```python
from build123d import *

# Parameters (mm, degrees)
F0_W     = 71
F0_H     = 7.4
F0_R     = 3
F1_DEPTH = 3.95
F0_R_2   = 2.499
F2_DEPTH = 2.95
F3_R     = 3.69999


# Not quite as in the source:
# - a fillet or chamfer is up to 0.001 mm smaller than in the source, because OpenCascade refuses the exact size


with BuildPart() as f1:
    # F0 (on Front) → F1 (new body, symmetric)
    with BuildSketch(Plane.XZ):
        Rectangle(F0_W, F0_H)
        with Locations((-32, 0)):
            Circle(F0_R, mode=Mode.SUBTRACT)
        with Locations((-24, 0)):
            Circle(F0_R, mode=Mode.SUBTRACT)
        with Locations((-16, 0)):
            Circle(F0_R, mode=Mode.SUBTRACT)
        with Locations((-8, 0)):
            Circle(F0_R, mode=Mode.SUBTRACT)
        Circle(F0_R, mode=Mode.SUBTRACT)
        with Locations((8, 0)):
            Circle(F0_R, mode=Mode.SUBTRACT)
        with Locations((16, 0)):
            Circle(F0_R, mode=Mode.SUBTRACT)
        with Locations((24, 0)):
            Circle(F0_R, mode=Mode.SUBTRACT)
        with Locations((32, 0)):
            Circle(F0_R, mode=Mode.SUBTRACT)
    extrude(amount=F1_DEPTH, both=True)

    # F0 (on Front) → F2 (join, symmetric)
    with BuildSketch(Plane.XZ):
        with Locations((-32, 0)):
            Circle(F0_R)
        with Locations((-32, 0)):
            Circle(F0_R_2, mode=Mode.SUBTRACT)
        with Locations((-24, 0)):
            Circle(F0_R)
        with Locations((-24, 0)):
            Circle(F0_R_2, mode=Mode.SUBTRACT)
        with Locations((-16, 0)):
            Circle(F0_R)
        with Locations((-16, 0)):
            Circle(F0_R_2, mode=Mode.SUBTRACT)
        with Locations((-8, 0)):
            Circle(F0_R)
        with Locations((-8, 0)):
            Circle(F0_R_2, mode=Mode.SUBTRACT)
        Circle(F0_R)
        Circle(F0_R_2, mode=Mode.SUBTRACT)
        with Locations((8, 0)):
            Circle(F0_R)
        with Locations((8, 0)):
            Circle(F0_R_2, mode=Mode.SUBTRACT)
        with Locations((16, 0)):
            Circle(F0_R)
        with Locations((16, 0)):
            Circle(F0_R_2, mode=Mode.SUBTRACT)
        with Locations((24, 0)):
            Circle(F0_R)
        with Locations((24, 0)):
            Circle(F0_R_2, mode=Mode.SUBTRACT)
        with Locations((32, 0)):
            Circle(F0_R)
        with Locations((32, 0)):
            Circle(F0_R_2, mode=Mode.SUBTRACT)
    extrude(amount=F2_DEPTH, both=True)

    # F3 (radius 3.7 in the source; OpenCascade refuses exactly that, so slightly less here)
    f3_edges = [f1.edges().sort_by_distance(p)[0] for p in [
        (-35.5, 0, 3.7),
        (-35.5, 0, -3.7),
        (35.5, 0, 3.7),
        (35.5, 0, -3.7),
    ]]
    fillet(f3_edges, radius=F3_R)


solid = f1.part
```
The listing builds one solid part. Answer for the finished solid, in the listing's coordinates (mm). A direction names the side the tool comes from. Give positions to 0.01 mm unless a question says otherwise; leave off trailing zeros. Order: outer loops, then holes, each group sorted by start corner. A loop starts at its lowest first (then second) coordinate and runs counter-clockwise, first axis right, second up. Notation, with made-up numbers: (86.25, 50) - (136.25, 50) arc R10 cw to (136.25, 65) - close; hole circle Ø4 at (45, 66). An arc over 180 degrees is marked (long way). Use one line per item in the form item = value. Start each with the question number.
(1) Consider line 1 (Z direction, x = -32, y = -2); line 2 (Z direction, x = 16, y = 3.2); line 3 (X direction, y = -2, z = 3.25). Determine where each line is inside the solid, lowest interval first. Write a range as from..to.
(2) A cutting plane is placed at B-B, the plane y = 1.5. State how many separate pieces and enclosed holes the cut face has, then the cut area to 3 significant figures.
(3) For faces 5 (the cylindrical face through (-34.44, 0.06, 2.59)), 6 (the cylindrical face through (-27, 3.5, 0.1)), 7 (the flat face through (14, -2.95, 2)), determine the directions among +Z, -Z, +X, -X, +Y, -Y from which every point of the face is accessible in a straight line to the end or side of a thin tool.
(4) The mould has two halves that part along Z. Classify faces 1 (the flat face through (0, 0, 3.7)), 2 (the cylindrical face through (10.77, 3.46, -1.15)), 3 (the flat face through (-26, -2.95, 2)), 4 (the flat face through (2.5, 3.95, -2.2)): released by +Z, released by -Z, zero draft, split by the parting line, or undercut.
(5) A cutting plane is placed at A-A, the plane x = 0. Write down the section's boundary in (y, z), then the cut area to 3 significant figures.
Ans:
q1.line_1 = -3.69..-2.5, 2.5..3.69
q1.line_2 = -3.7..-3, 3..3.7
q1.line_3 = -33.57..33.57
q2.separate_pieces = 1
q2.enclosed_holes = 9
q2.area = 337 mm^2
q3.face_5 = +Z, -X, +Y, -Y
q3.face_6 = +Y
q3.face_7 = -Y
q4.face_1 = released by +Z
q4.face_2 = undercut
q4.face_3 = undercut
q4.face_4 = zero draft
q5.outline = (-3.95, -3.7) - (3.95, -3.7) - (3.95, -3) - (2.95, -3) - (2.95, -2.5) - (-2.95, -2.5) - (-2.95, -3) - (-3.95, -3) - close; (-3.95, 3) - (-2.95, 3) - (-2.95, 2.5) - (2.95, 2.5) - (2.95, 3) - (3.95, 3) - (3.95, 3.7) - (-3.95, 3.7) - close
q5.area = 17.0 mm^2
